from build123d import *

# Parameters (mm, degrees)
SKETCH1_W            = 50.8
SKETCH1_H            = 50.038
BOSS_EXTRUDE1_DEPTH  = 1.27
SKETCH2_W            = 2.54
SKETCH2_H            = 30.48
BOSS_EXTRUDE2_DEPTH  = 11.43
SKETCH3_W            = 10.16
SKETCH3_H            = 20.32
BOSS_EXTRUDE3_DEPTH  = 3.81
SKETCH4_W            = 50.8
SKETCH4_H            = 50.038
BOSS_EXTRUDE4_DEPTH  = 1.27
SKETCH5_W            = 10.16
SKETCH5_H            = 38.1
SKETCH5_W_2          = 15.24
SKETCH5_H_2          = 2.54
SKETCH5_W_3          = 5.08
BOSS_EXTRUDE5_DEPTH  = 7.874
SKETCH5_3_W          = 5.08
SKETCH5_3_H          = 5.08
BOSS_EXTRUDE6_DEPTH  = 3.175
SKETCH5_4_R          = 1.397
BOSS_EXTRUDE7_DEPTH  = 5.08
SKETCH5_5_W          = 11.43
SKETCH5_5_H          = 3.175
BOSS_EXTRUDE8_DEPTH  = 6.35
BOSS_EXTRUDE9_DEPTH  = 3.81
FILLET1_R            = 1.27
SKETCH8_R            = 1.5875
BOSS_EXTRUDE10_DEPTH = 0.635
SKETCH9_W            = 2.427127008
SKETCH9_H            = 1.995592696
BOSS_EXTRUDE11_DEPTH = 2.54


with BuildPart() as part:
    # Sketch1 → Boss-Extrude1 (new body)
    with BuildSketch(Plane(origin=(0, 0, 0), x_dir=(1, 0, 0), z_dir=(0, 1, 0))):
        Rectangle(SKETCH1_W, SKETCH1_H)
    extrude(amount=BOSS_EXTRUDE1_DEPTH)

    # Sketch2 → Boss-Extrude2 (add)
    with BuildSketch(Plane(origin=(0, 1.27, 0), x_dir=(1, 0, 0), z_dir=(0, 1, 0))):
        with Locations((-22.352, -3.175)):
            Rectangle(SKETCH2_W, SKETCH2_H)
        with Locations((22.352, -3.175)):
            Rectangle(SKETCH2_W, SKETCH2_H)
    extrude(amount=BOSS_EXTRUDE2_DEPTH)

    # Sketch3 → Boss-Extrude3 (add)
    with BuildSketch(Plane(origin=(0, 1.27, 0), x_dir=(1, 0, 0), z_dir=(0, 1, 0))):
        with Locations((0, 13.335)):
            Rectangle(SKETCH3_W, SKETCH3_H)
    extrude(amount=BOSS_EXTRUDE3_DEPTH)

    # Sketch4 → Boss-Extrude4 (add)
    with BuildSketch(Plane(origin=(0, 12.7, 0), x_dir=(1, 0, 0), z_dir=(0, 1, 0))):
        Rectangle(SKETCH4_W, SKETCH4_H)
    extrude(amount=BOSS_EXTRUDE4_DEPTH)

    # Sketch5 → Boss-Extrude5 (add)
    with BuildSketch(Plane(origin=(0, 13.97, 0), x_dir=(1, 0, 0), z_dir=(0, 1, 0))):
        with Locations((0, -0.889)):
            Rectangle(SKETCH5_W, SKETCH5_H)
        with Locations((-9.966399328, 22.733)):
            Rectangle(SKETCH5_W_2, SKETCH5_H_2)
        with Locations((-21.396399328, 22.733)):
            Rectangle(SKETCH5_W_3, SKETCH5_H_2)
    extrude(amount=BOSS_EXTRUDE5_DEPTH)

    # Sketch5_3 → Boss-Extrude6 (add)
    with BuildSketch(Plane(origin=(0, 13.97, 0), x_dir=(1, 0, 0), z_dir=(0, 1, 0))):
        with Locations((-16.51, -21.209)):
            Rectangle(SKETCH5_3_W, SKETCH5_3_H)
        with Locations((-10.922, -21.209)):
            Rectangle(SKETCH5_3_W, SKETCH5_3_H)
    extrude(amount=BOSS_EXTRUDE6_DEPTH)

    # Sketch5_4 → Boss-Extrude7 (add)
    with BuildSketch(Plane(origin=(0, 13.97, 0), x_dir=(1, 0, 0), z_dir=(0, 1, 0))):
        with Locations((13.16676441, -21.867024383)):
            Circle(SKETCH5_4_R)
        with Locations((17.978093258, -21.867024383)):
            Circle(SKETCH5_4_R)
        with Locations((15.135118943, 17.046813881)):
            Circle(SKETCH5_4_R)
    extrude(amount=BOSS_EXTRUDE7_DEPTH)

    # Sketch5_5 → Boss-Extrude8 (add)
    with BuildSketch(Plane(origin=(0, 13.97, 0), x_dir=(1, 0, 0), z_dir=(0, 1, 0))):
        with Locations((8.448600672, 22.733)):
            Rectangle(SKETCH5_5_W, SKETCH5_5_H)
    extrude(amount=BOSS_EXTRUDE8_DEPTH)

    # Sketch5_6 → Boss-Extrude9 (add)
    with BuildSketch(Plane(origin=(0, 13.97, 0), x_dir=(1, 0, 0), z_dir=(0, 1, 0))):
        with BuildLine():
            Line((20.260877265, 24.3205), (24.356504201, 24.3205))
            ThreePointArc((24.356504201, 24.3205), (22.308690733, 21.0185), (20.260877265, 24.3205))
        make_face()
    extrude(amount=BOSS_EXTRUDE9_DEPTH)

    # Fillet1
    fillet1_edges = [part.edges().sort_by_distance(p)[0] for p in [
        (11.76976441, 19.05, 21.867024383),
        (16.581093258, 19.05, 21.867024383),
        (13.738118943, 19.05, -17.046813881),
    ]]
    fillet(fillet1_edges, radius=FILLET1_R)

    # Sketch8 → Boss-Extrude10 (add)
    with BuildSketch(Plane(origin=(0, 17.145, 0), x_dir=(1, 0, 0), z_dir=(0, 1, 0))):
        with Locations((-16.51, -21.209)):
            Circle(SKETCH8_R)
        with Locations((-10.922, -21.209)):
            Circle(SKETCH8_R)
    extrude(amount=BOSS_EXTRUDE10_DEPTH)

    # Sketch9 → Boss-Extrude11 (add)
    with BuildSketch(Plane(origin=(0, 20.32, 0), x_dir=(1, 0, 0), z_dir=(0, 1, 0))):
        with Locations((11.306100672, 22.733)):
            Rectangle(SKETCH9_W, SKETCH9_H)
    extrude(amount=BOSS_EXTRUDE11_DEPTH)


solid = part.part
Input: part model. Units: mm. Frame: model coordinates. A direction names the side the tool comes from. Coordinates: 2 decimals unless noted, no trailing zeros. Loops run counter-clockwise (first coordinate to the right, second up) from the corner with the lowest first, then second, coordinate; pieces in that order, holes last. Notation, with made-up numbers: (-31.5, 30.5) - (-7.5, 30.5) arc R20 cw to (-7.5, 35.5) - close; hole circle Ø6 at (5, 19.25). An arc over 180 degrees is marked (long way). Answer in a Markdown table with one row per item. Add a question column.
Item 1: Section query D-D on y = 15.25. State how many separate pieces and enclosed holes the cut face has, then the cut area to 3 significant figures.
Item 2: Section query A-A on y = 3.5. Return the cut outline in (x, z) (3 decimals), then the cut area to 3 significant figures.
Item 3: Line query: line 1 along X through (y, z) = (1.75, -9); line 2 along Y through (x, z) = (-6.5, 16.5); line 3 along X through (y, z) = (11, 10). Output: solid intervals per line, ascending. Write a range as [from, to].
Item 4: Section query C-C on x = -16.51. Return the cut outline in (y, z) (1 decimal).
Item 5: Section query B-B on z = -6. Return the cut outline in (x, y).
Item 6: Mould query, pull axis Z, two halves, no side actions, for faces 6 (the flat face through (12.52, 22, -23)), 7 (the flat face through (0, 1, -25.019)), 8 (the flat face through (5.3, 13.97, -0.4)). Classes: released by +Z, released by -Z, zero draft, split by the parting line, or undercut.
Item 7: Access query for faces 1 (the flat face through (-17.586, 18, -23)), 2 (the flat face through (-11, 16, 23.749)), 3 (the flat face through (-18, 17.145, 20)), 4 (the flat face through (-11, 17.78, 21)), 5 (the flat face through (21.082, 7, 3)). Directions: +Z, -Z, +X, -X, +Y, -Y. A direction counts if a zero-diameter tool reaches every point of the face in a straight line with its end or side. Return the directions, or none.
Item 8: Contact query for flat-ended pins moving along their axis: P1, Ø1.5, axis at y = 6.5, z = 0, coming from the -X side; P2, Ø8, axis at x = 1, z = -8.5, coming from the +Y side; P3, Ø0.6, axis at y = 21.5, z = -23, coming from the +X side; P4, Ø9, axis at y = 5.5, z = 10, coming from the -X side. Output: stop coordinate, or through.
Recorded:
| question | item | result |
|---|---|---|
| 1 | separate pieces | 10 |
| 1 | enclosed holes | 0 |
| 1 | area | 558 mm^2 |
| 2 | outline | (-23.622, -12.065) - (-21.082, -12.065) - (-21.082, 18.415) - (-23.622, 18.415) - close; (-5.08, -23.495) - (5.08, -23.495) - (5.08, -3.175) - (-5.08, -3.175) - close; (21.082, -12.065) - (23.622, -12.065) - (23.622, 18.415) - (21.082, 18.415) - close |
| 2 | area | 361 mm^2 |
| 3 | line 1 | [-23.62, -21.08], [-5.08, 5.08], [21.08, 23.62] |
| 3 | line 2 | [0, 1.27], [12.7, 13.97] |
| 3 | line 3 | [-23.62, -21.08], [21.08, 23.62] |
| 4 | outline | (0, -25) - (1.3, -25) - (1.3, 25) - (0, 25) - close; (12.7, -25) - (14, -25) - (14, -24) - (21.8, -24) - (21.8, -21.5) - (14, -21.5) - (14, 18.7) - (17.1, 18.7) - (17.1, 19.6) - (17.8, 19.6) - (17.8, 22.8) - (17.1, 22.8) - (17.1, 23.7) - (14, 23.7) - (14, 25) - (12.7, 25) - close |
| 5 | outline | (-25.4, 0) - (25.4, 0) - (25.4, 1.27) - (23.62, 1.27) - (23.62, 12.7) - (25.4, 12.7) - (25.4, 13.97) - (5.08, 13.97) - (5.08, 21.84) - (-5.08, 21.84) - (-5.08, 13.97) - (-25.4, 13.97) - (-25.4, 12.7) - (-23.62, 12.7) - (-23.62, 1.27) - (-25.4, 1.27) - close; hole (-21.08, 1.27) - (-5.08, 1.27) - (-5.08, 5.08) - (5.08, 5.08) - (5.08, 1.27) - (21.08, 1.27) - (21.08, 12.7) - (-21.08, 12.7) - close |
| 6 | face 6 | zero draft |
| 6 | face 7 | released by -Z |
| 6 | face 8 | undercut |
| 7 | face 1 | -Z, +Y |
| 7 | face 2 | +Z, +X, -X, +Y |
| 7 | face 3 | +Y |
| 7 | face 4 | +Z, -X, +Y |
| 7 | face 5 | +Z, -Z |
| 8 | P1 | x = -23.62 |
| 8 | P2 | y = 21.84 |
| 8 | P3 | x = 12.52 |
| 8 | P4 | x = -25.4 |
